Read the model definition and answer for the solid it produces. Units are mm, in the model's axes. A direction names the side the tool comes from. Coordinates: 2 decimals unless noted, no trailing zeros. Write each loop counter-clockwise with the first axis right and the second up, starting at its lowest first coordinate (ties: lowest second). Pieces come first, ordered by that corner, then holes.
(1) Straight lines are drawn through the part: line 1 along Y through (x, z) = (0, 6.05); line 2 along X through (y, z) = (-0.5, 5); line 3 along Z through (x, y) = (16.5, 4). For each, find the intervals that lie inside material, in ascending order.
(2) The part is cut by section A-A, the plane x = 0. State how many separate pieces and enclosed holes the cut face has, and give its area (3 significant figures).
(3) The part is cut by section B-B, the plane z = 5.5. Determine the outline of the cut face in (x, y), and give its area (3 significant figures).
(4) The part is cut by section D-D, the plane y = 17.5. Determine the outline of the cut face in (x, z), and give its area (3 significant figures).
(5) Determine the mould class of faces 4 (the flat face through (-12.514, 12.234, 3.451)), 5 (the flat face through (12.514, -12.234, 3.451)), 6 (the cylindrical face through (-22.5, 0, 3.5)), 7 (the cylindrical face through (0.488, -19.696, 5.479)) for opening direction Y: pulls with the +Y half, pulls with the -Y half, needs draft (parallel to the pull), parting line crosses it, or undercut.
(6) Which of the six approach directions +Z, -Z, +X, -X, +Y, -Y give full straight-line access (tool end or side, diameter ignored) to faces 1 (the flat face through (15.1, 1.8, 7)), 2 (the cylindrical face through (0.423, 20.722, 1.972)), 3 (the cylindrical face through (-0.867, -3.905, 5.577))?
(7) Given pin 1 (3 mm diameter, centred on y = -2, z = 1.5, fed in from -X); pin 2 (3 mm diameter, centred on x = -1, y = -17, fed in from -Z); pin 3 (1 mm diameter, centred on x = -17, z = 6.5, fed in from -Y), each flat-ended and moving along its own axis, determine where each tip first touches the part or whether it passes through.
```python
from build123d import *

# Parameters (mm, degrees)
BOSS_EXTRUDE1_DEPTH = 7
SKETCH2_R           = 3.25
CUT_EXTRUDE1_DEPTH  = 4
SKETCH3_R           = 1.7
SKETCH3_R_2         = 2.25
CUT_EXTRUDE2_DEPTH  = 4
SKETCH4_R           = 14
BOSS_EXTRUDE2_DEPTH = 5
SKETCH5_R           = 4
CUT_EXTRUDE3_DEPTH  = 15
FILLET3_R           = 1


with BuildPart() as part:
    # Sketch1 → Boss-Extrude1 (new body)
    with BuildSketch(Plane.XY):
        with BuildLine():
            Line((-12.374368671, -12.374368671), (-22.374368671, -2.374368671))
            ThreePointArc((-22.374368671, -2.374368671), (-22.5, 0), (-22.374368671, 2.374368671))
            Line((-22.374368671, 2.374368671), (-12.374368671, 12.374368671))
            Line((-12.374368671, 12.374368671), (-2.374368671, 22.374368671))
            ThreePointArc((-2.374368671, 22.374368671), (0, 22.5), (2.374368671, 22.374368671))
            Line((2.374368671, 22.374368671), (12.374368671, 12.374368671))
            Line((12.374368671, 12.374368671), (22.374368671, 2.374368671))
            ThreePointArc((22.374368671, 2.374368671), (22.5, 0), (22.374368671, -2.374368671))
            Line((22.374368671, -2.374368671), (12.374368671, -12.374368671))
            Line((12.374368671, -12.374368671), (2.374368671, -22.374368671))
            ThreePointArc((2.374368671, -22.374368671), (0, -22.5), (-2.374368671, -22.374368671))
            Line((-2.374368671, -22.374368671), (-12.374368671, -12.374368671))
        make_face()
    extrude(amount=BOSS_EXTRUDE1_DEPTH)

    # Sketch2 → Cut-Extrude1 (cut)
    with BuildSketch(Plane(origin=(0, 0, 0), x_dir=(-1, 0, 0), z_dir=(0, 0, -1))):
        with Locations((0, 17.5)):
            Circle(SKETCH2_R)
        with Locations((-17.5, 0)):
            Circle(SKETCH2_R)
        with Locations((0, -17.5)):
            Circle(SKETCH2_R)
        with Locations((17.5, 0)):
            Circle(SKETCH2_R)
    extrude(amount=-CUT_EXTRUDE1_DEPTH, mode=Mode.SUBTRACT)

    # Sketch3 → Cut-Extrude2 (cut)
    with BuildSketch(Plane(origin=(0, 0, 4), x_dir=(-1, 0, 0), z_dir=(0, 0, -1))):
        with Locations((0, 17.5)):
            Circle(SKETCH3_R)
        with Locations((-17.5, 0)):
            Circle(SKETCH3_R_2)
        with Locations((17.5, 0)):
            Circle(SKETCH3_R_2)
        with Locations((0, -17.5)):
            Circle(SKETCH3_R_2)
    extrude(amount=-CUT_EXTRUDE2_DEPTH, mode=Mode.SUBTRACT)

    # Sketch4 → Boss-Extrude2 (add)
    with BuildSketch(Plane.XY.offset(7)):
        Circle(SKETCH4_R)
    extrude(amount=BOSS_EXTRUDE2_DEPTH)

    # Sketch5 → Cut-Extrude3 (cut)
    with BuildSketch(Plane.XY.offset(12)):
        Circle(SKETCH5_R)
    extrude(amount=-CUT_EXTRUDE3_DEPTH, mode=Mode.SUBTRACT)

    # Fillet3
    fillet3_edges = [part.edges().sort_by_distance(p)[0] for p in [
        (-14, 0, 7),
        (-14, 0, 12),
        (-4, 0, 12),
    ]]
    fillet(fillet3_edges, radius=FILLET3_R)


solid = part.part
```
Computed:
1. line 1: y = -22.5 to -19.75, -15.25 to -4, 4 to 15.8, 19.2 to 22.5
1. line 2: x = -22.49 to -19.69, -15.31 to -3.97, 3.97 to 15.31, 19.69 to 22.49
1. line 3: z = 0 to 7
2. separate pieces: 4
2. enclosed holes: 0
2. area: 283 mm2
3. outline: (-22.37, -2.37) - (-2.37, -22.37) arc R22.5 ccw to (2.37, -22.37) - (22.37, -2.37) arc R22.5 ccw to (22.37, 2.37) - (2.37, 22.37) arc R22.5 ccw to (-2.37, 22.37) - (-22.37, 2.37) arc R22.5 ccw to start; hole circle Ø4.5 at (-17.5, 0); hole circle Ø8 at (0, 0); hole circle Ø4.5 at (0, -17.5); hole circle Ø3.4 at (0, 17.5); hole circle Ø4.5 at (17.5, 0)
3. area: 1,100 mm2
4. outline: (-7.25, 0) - (-3.25, 0) - (-3.25, 4) - (-1.7, 4) - (-1.7, 7) - (-7.25, 7) - close; (1.7, 4) - (3.25, 4) - (3.25, 0) - (7.25, 0) - (7.25, 7) - (1.7, 7) - close
4. area: 65.3 mm2
5. face 4: pulls with the +Y half
5. face 5: pulls with the -Y half
5. face 6: parting line crosses it
5. face 7: undercut
6. face 1: +Z
6. face 2: -Z
6. face 3: +Z, -Z
7. pin 1: stops at x = -22.49
7. pin 2: stops at z = 4
7. pin 3: stops at y = -8.25
